from build123d import *

# Parameters (mm, degrees)
SKETCH1_W            = 22.6
SKETCH1_H            = 11.84
BOSS_EXTRUDE1_DEPTH  = 22.7
SKETCH4_R            = 5.84
BOSS_EXTRUDE6_DEPTH  = 4.5
SKETCH12_R           = 2.335
BOSS_EXTRUDE7_DEPTH  = 2.5
SKETCH13_R           = 2.5
BOSS_EXTRUDE8_DEPTH  = 4.5
SKETCH14_W           = 11.84
SKETCH14_H           = 2.37
BOSS_EXTRUDE10_DEPTH = 4.5
SKETCH15_R           = 1
SKETCH15_W           = 1.5
SKETCH15_H           = 1
CUT_EXTRUDE3_DEPTH   = 51.362478675
SKETCH16_W           = 11.84
SKETCH16_H           = 2.37
BOSS_EXTRUDE11_DEPTH = 4.5
SKETCH17_R           = 1
SKETCH17_W           = 1.5
SKETCH17_H           = 1
CUT_EXTRUDE4_DEPTH   = 55.51962078
SKETCH18_R           = 2.5
CUT_EXTRUDE5_DEPTH   = 3


with BuildPart() as part:
    # Sketch1 → Boss-Extrude1 (new body)
    with BuildSketch(Plane(origin=(0, 0, 0), x_dir=(1, 0, 0), z_dir=(0, 1, 0))):
        with Locations((-34.895532414, -1.336861806)):
            Rectangle(SKETCH1_W, SKETCH1_H)
    extrude(amount=BOSS_EXTRUDE1_DEPTH)

    # Sketch4 → Boss-Extrude6 (add)
    with BuildSketch(Plane(origin=(0, 22.7, 0), x_dir=(-1, 0, 0), z_dir=(0, 1, 0))):
        with Locations((40.355532414, 1.336861806)):
            Circle(SKETCH4_R)
    extrude(amount=BOSS_EXTRUDE6_DEPTH)

    # Sketch12 → Boss-Extrude7 (add)
    with BuildSketch(Plane(origin=(0, 27.2, 0), x_dir=(-1, 0, 0), z_dir=(0, 1, 0))):
        with Locations(Location((40.355532414, 1.336861806, 0), (0, 0, 90))):
            Circle(SKETCH12_R)
    extrude(amount=BOSS_EXTRUDE7_DEPTH)

    # Sketch13 → Boss-Extrude8 (add)
    with BuildSketch(Plane(origin=(0, 22.7, 0), x_dir=(-1, 0, 0), z_dir=(0, 1, 0))):
        with Locations((34.015532414, 1.336861806)):
            Circle(SKETCH13_R)
    extrude(amount=BOSS_EXTRUDE8_DEPTH)

    # Sketch14 → Boss-Extrude10 (add)
    with BuildSketch(Plane(origin=(-23.595532414, 0, 0), x_dir=(0, 0, -1), z_dir=(1, 0, 0))):
        with Locations((-1.336861806, 17.515)):
            Rectangle(SKETCH14_W, SKETCH14_H)
    extrude(amount=BOSS_EXTRUDE10_DEPTH)

    # Sketch15 → Cut-Extrude3 (cut, through all)
    with BuildSketch(Plane(origin=(0, 18.7, 0), x_dir=(-1, 0, 0), z_dir=(0, 1, 0))):
        with Locations((21.395532414, 1.336861806)):
            Circle(SKETCH15_R)
        with Locations((48.395532414, 1.336861806)):
            Circle(SKETCH15_R)
        with Locations((19.845532414, 1.336861806)):
            Rectangle(SKETCH15_W, SKETCH15_H)
    extrude(amount=-CUT_EXTRUDE3_DEPTH, mode=Mode.SUBTRACT)

    # Sketch16 → Boss-Extrude11 (add)
    with BuildSketch(Plane.ZY.offset(46.195532414)):
        with Locations((1.336861806, 17.515)):
            Rectangle(SKETCH16_W, SKETCH16_H)
    extrude(amount=BOSS_EXTRUDE11_DEPTH)

    # Sketch17 → Cut-Extrude4 (cut, through all)
    with BuildSketch(Plane(origin=(0, 18.7, 0), x_dir=(-1, 0, 0), z_dir=(0, 1, 0))):
        with Locations((48.295532414, 1.336861806)):
            Circle(SKETCH17_R)
        with Locations((49.945532414, 1.336861806)):
            Rectangle(SKETCH17_W, SKETCH17_H)
    extrude(amount=-CUT_EXTRUDE4_DEPTH, mode=Mode.SUBTRACT)

    # Sketch18 → Cut-Extrude5 (cut)
    with BuildSketch(Plane(origin=(0, 0, 0), x_dir=(-1, 0, 0), z_dir=(0, -1, 0))):
        with Locations(Location((40.355532414, -1.336861806, 0), (0, 0, 90))):
            Circle(SKETCH18_R)
    extrude(amount=-CUT_EXTRUDE5_DEPTH, mode=Mode.SUBTRACT)


solid = part.part
Build history of the part. All positions in model axes, mm. A direction names the side the tool comes from. Coordinates: 2 decimals unless noted, no trailing zeros. Order: outer loops, then holes, each group sorted by start corner. A loop starts at its lowest first (then second) coordinate and runs counter-clockwise, first axis right, second up. Notation, with made-up numbers: M -0.5,-3.75 L 49.5,-3.75 A36 cw 49.5,35.25 Z; hole C 81.5,77 d8. An arc over 180 degrees is marked long. One line per question, with ' | ' between items. Start each with the question number.
Q1. Saw through at C-C (z = 4.5). List the corners of the cut face in (x, y).
Q2. Saw through at D-D (x = -41.5). List the corners of the cut face in (y, z), then the cut area to 3 significant figures.
Q3. Saw through at B-B (x = -21.5). List the corners of the cut face in (y, z).
Q4. Saw through at A-A (y = 18.25). List the corners of the cut face in (x, z).
Q5. Two-plate mould, pull along Z, no slides. Class faces 4 (the face through (-20, 18, 0.837)), 5 (the face through (-46.19, 24.92, 1.11)), 6 (the face through (-46.196, 21, 1)): +Z half, -Z half, draft (parallel to the pull), parting line (faces both ways), or undercut.
Q6. Probe L1, parallel to Y at x = -46.5, z = 3.5; L2, parallel to Y at x = -43.5, z = 6.5; L3, parallel to X at y = 10.75, z = -3. List the from-to ranges inside material, lowest first. Write a range as from..to.
Q7. 3-axis set-ups, long thin cutter, end or side, ignore diameter. For faces 1 (the face through (-21, 18.7, 3)), 2 (the face through (-48, 18.7, 3)), 3 (the face through (-37, 27.2, 1)): which of +Z, -Z, +X, -X, +Y, -Y reach the whole face in a straight line?
Q8. Flat gauge pins, fed straight in: pin 1 Ø1.3 at (x, z) = (-21, 4) entering from -Y; pin 2 Ø4 at (y, z) = (11, -1) entering from -X; pin 3 Ø1 at (y, z) = (8, -1.5) entering from +X. Where does each tip first touch, or does it go through?
Check values:
1) outline: M -50.7,16.33 L -46.2,16.33 L -46.2,0 L -23.6,0 L -23.6,16.33 L -19.1,16.33 L -19.1,18.7 L -23.6,18.7 L -23.6,22.7 L -35.45,22.7 L -35.45,27.2 L -45.26,27.2 L -45.26,22.7 L -46.2,22.7 L -46.2,18.7 L -50.7,18.7 Z
2) outline: M 0,-4.58 L 22.7,-4.58 L 22.7,-4.39 L 27.2,-4.39 L 27.2,-0.7 L 29.7,-0.7 L 29.7,3.37 L 27.2,3.37 L 27.2,7.06 L 22.7,7.06 L 22.7,7.26 L 0,7.26 L 0,3.56 L 3,3.56 L 3,-0.89 L 0,-0.89 Z | area: 317 mm2
3) outline: M 16.33,-4.58 L 18.7,-4.58 L 18.7,0.34 L 16.33,0.34 Z; M 16.33,2.33 L 18.7,2.33 L 18.7,7.26 L 16.33,7.26 Z
4) outline: M -50.7,-4.58 L -19.1,-4.58 L -19.1,0.84 L -20.53,0.84 A1 cw long -20.53,1.84 L -19.1,1.84 L -19.1,7.26 L -50.7,7.26 L -50.7,1.84 L -49.2,1.84 L -49.2,1.77 A1 cw long -49.2,0.9 L -49.2,0.84 L -50.7,0.84 Z
5) face 4: undercut | face 5: parting line | face 6: draft
6) L1: y = 16.33..18.7 | L2: y = 0..22.7 | L3: x = -46.2..-23.6
7) face 1: +Z, -Z, +X, +Y | face 2: +Z, -Z, -X, +Y | face 3: +Y
8) pin 1: stops at y = 16.33 | pin 2: stops at x = -46.2 | pin 3: stops at x = -23.6
